Answer from the drawing. Dimensions are ordinates in mm from the lowest x, y and z of the part. Round coordinates to 2 decimals unless told otherwise and drop trailing zeros. Write each loop counter-clockwise with the first axis right and the second up, starting at its lowest first coordinate (ties: lowest second). Pieces come first, ordered by that corner, then holes. Notation, with made-up numbers: (47, -40) -> (77, -40) arc R29 cw to (77, -14) -> close; hole circle Ø5 at (-21, 52.25). An arc over 180 degrees is marked (long way). Return JSON: item names as keys, results as strings. Group by question number.
(1) A cutting plane is placed at A-A on x = 27. Give the vertices of the cut face in (y, z) (3 decimals).
(2) Straight lines are drawn through the part: line 1 (Y direction, x = 17, z = 1.45) (3 decimals); line 2 (Z direction, x = 27, y = 5) (3 decimals); line 3 (Z direction, x = 75, y = 4.25) (3 decimals). For each, find the intervals that lie inside material, in ascending order.
(3) The mould has two halves that part along X. Classify the marked faces 1, 2 and 3: released by +X, released by -X, zero draft, split by the parting line, or undercut.
(4) A cutting plane is placed at D-D on y = 5.5. Give the vertices of the cut face in (x, z) (3 decimals), then the cut area to 3 significant figures.
(5) A cutting plane is placed at C-C on x = 17. Give the vertices of the cut face in (y, z) (3 decimals), then the cut area to 3 significant figures.
(6) Given pin 1 (0.9 mm diameter, centred on x = 68.5, y = 2.5, fed in from -Z), flat-ended and moving along its own axis, determine where the tip first touches the part or whether it passes through.
(7) A cutting plane is placed at B-B on z = 6. Give the vertices of the cut face in (x, y).
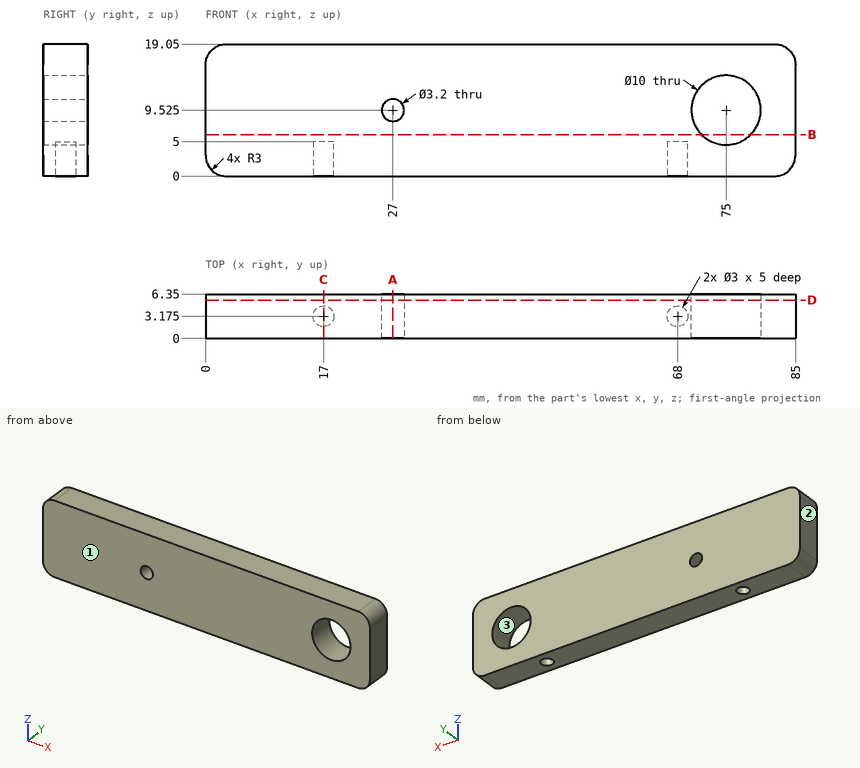
Checks:
{
 "1": {"outline": "(0, 0) -> (6.35, 0) -> (6.35, 7.925) -> (0, 7.925) -> close; (0, 11.125) -> (6.35, 11.125) -> (6.35, 19.05) -> (0, 19.05) -> close"},
 "2": {"line 1": "y = 0 to 1.675, 4.675 to 6.35", "line 2": "z = 0 to 7.925, 11.125 to 19.05", "line 3": "z = 0 to 4.525, 14.525 to 19.05"},
 "3": {"face 1": "zero draft", "face 2": "released by -X", "face 3": "undercut"},
 "4": {"outline": "(0, 3) arc R3 ccw to (3, 0) -> (82, 0) arc R3 ccw to (85, 3) -> (85, 16.05) arc R3 ccw to (82, 19.05) -> (3, 19.05) arc R3 ccw to (0, 16.05) -> close; hole circle Ø3.2 at (27, 9.525); hole circle Ø10 at (75, 9.525)", "area": "1,520 mm^2"},
 "5": {"outline": "(0, 0) -> (1.675, 0) -> (1.675, 5) -> (4.675, 5) -> (4.675, 0) -> (6.35, 0) -> (6.35, 19.05) -> (0, 19.05) -> close", "area": "106 mm^2"},
 "6": {"pin 1": "stops at z = 5"},
 "7": {"outline": "(0, 0) -> (71.45, 0) -> (71.45, 6.35) -> (0, 6.35) -> close; (78.55, 0) -> (85, 0) -> (85, 6.35) -> (78.55, 6.35) -> close"}
}
